The listing builds one solid part. Answer for the finished solid, in the listing's coordinates (mm). A direction names the side the tool comes from. Round coordinates to 2 decimals unless told otherwise and drop trailing zeros. Write each loop counter-clockwise with the first axis right and the second up, starting at its lowest first coordinate (ties: lowest second). Pieces come first, ordered by that corner, then holes. Notation, with made-up numbers: M -1,22 L 30,22 A37 cw 30,60 Z; hole C 18,26.25 d10. An arc over 180 degrees is marked long. One line per item, written item: value. Start each with the question number.
(1) Section A-A (y = 1.5) is taken. Determine the outline of the cut face in (x, z).
(2) Section C-C (z = 3.25) is taken. Determine the outline of the cut face in (x, y), plus the area to 3 significant figures.
(3) Consider probe 1 along X at (y, z) = (5.25, 4.2); probe 2 along X at (y, z) = (4.5, 3.55); probe 3 along Y at (x, z) = (3.75, 1.1). Determine where each line is inside the solid, lowest interval first.
(4) Section D-D (x = 0) is taken. Determine the outline of the cut face in (y, z), plus the area to 3 significant figures.
(5) For faces 4 (the flat face through (4.5, 2.6, 2.5)), 5 (the flat face through (-4, 5, 2)), 6 (the flat face through (-3, 3, 2)), 7 (the flat face through (3.5, 4, 2)), determine the directions among +Z, -Z, +X, -X, +Y, -Y from which every point of the face is accessible in a straight line to the end or side of a thin tool.
(6) For a pull along Y with two mould halves and no side action, classify faces 1 (the flat face through (-3.5, 4, 2)), 2 (the cylindrical face through (0, -3, 2)), 3 (the flat face through (-4.5, 2.6, 2.5)) as released by +Y, released by -Y, zero draft, split by the parting line, or undercut.
(7) Section B-B (x = 4) is taken. Determine the outline of the cut face in (y, z).
(8) Given P1, Ø3, axis at x = -0.5, z = 3, coming from the -Y side; P2, Ø1.1, axis at x = -4, z = 2, coming from the -Y side; P3, Ø0.6, axis at y = 5.5, z = 3, coming from the -X side; P4, Ø0.8, axis at x = -4, z = 3.5, coming from the +Y side, each flat-ended and moving along its own axis, determine where each tip first touches the part or whether it passes through.
```python
from build123d import *

# Parameters (mm, degrees)
F1_DEPTH = 5


with BuildPart() as f1:
    # F0 (on Top) → F1 (new body)
    with BuildSketch(Plane.XY):
        with BuildLine():
            Line((-4.5, 3), (-4.5, 2.179449))
            ThreePointArc((-4.5, 2.179449), (0, -5), (4.5, 2.179449))
            Line((4.5, 2.179449), (4.5, 3))
            Line((4.5, 3), (3.5, 3))
            Line((3.5, 3), (3.5, 5))
            Line((3.5, 5), (4.5, 5))
            Line((4.5, 5), (4.5, 5.5))
            Line((4.5, 5.5), (3, 6))
            Line((3, 6), (3, 0))
            ThreePointArc((3, 0), (0, -3), (-3, 0))
            Line((-3, 0), (-3, 6))
            Line((-3, 6), (-4.5, 5.5))
            Line((-4.5, 5.5), (-4.5, 5))
            Line((-4.5, 5), (-3.5, 5))
            Line((-3.5, 5), (-3.5, 3))
            Line((-3.5, 3), (-4.5, 3))
        make_face()
    extrude(amount=F1_DEPTH)


solid = f1.part
```
Recorded:
1. outline: M -4.77,0 L -3,0 L -3,5 L -4.77,5 Z; M 3,0 L 4.77,0 L 4.77,5 L 3,5 Z
2. outline: M -4.5,2.18 A5 ccw long 4.5,2.18 L 4.5,3 L 3.5,3 L 3.5,5 L 4.5,5 L 4.5,5.5 L 3,6 L 3,0 A3 cw -3,0 L -3,6 L -4.5,5.5 L -4.5,5 L -3.5,5 L -3.5,3 L -4.5,3 Z
2. area: 39.9 mm2
3. probe 1: x = -4.5 to -3, 3 to 4.5
3. probe 2: x = -3.5 to -3, 3 to 3.5
3. probe 3: y = -3.31 to 3, 5 to 5.75
4. outline: M -5,0 L -3,0 L -3,5 L -5,5 Z
4. area: 10.0 mm2
5. face 4: +Z, -Z, +X, +Y
5. face 5: +Z, -Z, -X
5. face 6: +Z, -Z, +Y
5. face 7: +Z, -Z, +X
6. face 1: undercut
6. face 2: released by +Y
6. face 3: zero draft
7. outline: M -3,0 L 3,0 L 3,5 L -3,5 Z; M 5,0 L 5.67,0 L 5.67,5 L 5,5 Z
8. P1: stops at y = -5
8. P2: stops at y = -3.62
8. P3: stops at x = -4.5
8. P4: stops at y = 5.8
